Design review of the part shown in the three views and the two pictorial views. Dimensions are in mm from the part's minimum x, y and z. Coordinates: 2 decimals unless noted, no trailing zeros. Loops run counter-clockwise (first coordinate to the right, second up) from the corner with the lowest first, then second, coordinate; pieces in that order, holes last. Notation, with made-up numbers: M 41,-37 L 73,-37 A20 ccw 73,-1 Z; hole C 49.5,41.5 d8. An arc over 180 degrees is marked long. Answer as a JSON object with one key per item and string values. Group by question number.
Item 1: Wall thickness on L1, parallel to X at y = 1.7, z = 3; L2, parallel to X at y = 1.55, z = 3.5; L3, parallel to X at y = 0.4, z = 9: over which ranges is each line inside the solid? List them lowest first. Write a range as from..to.
Item 2: Add section D-D (y = 0.9). State the section outline as (x, z) points.
Item 3: Add section B-B (z = 7). State the section outline as (x, y) points (3 decimals), then the cut area to 3 significant figures.
Item 4: Insertion check: pin 1 (1.8 mm diameter, centred on x = 3, z = 3, fed in from -Y); pin 2 (6 mm diameter, centred on x = 4, z = 2.5, fed in from -Y). Each pin has a flat end and moves straight along its axis. Give the tip position at first contact, or say it passes through.
Item 5: Add section C-C (x = 17). State the section outline as (y, z) points, then the cut area to 3 significant figures.
Item 6: Add section A-A (y = 3.3). State the section outline as (x, z) points, then the cut area to 3 significant figures.
Item 7: Mouldability with a two-part tool opening along Z and no side actions: class the marked faces 1, 2, 3 and 4 as +Z half, -Z half, draft (parallel to the pull), parting line (faces both ways), or undercut.
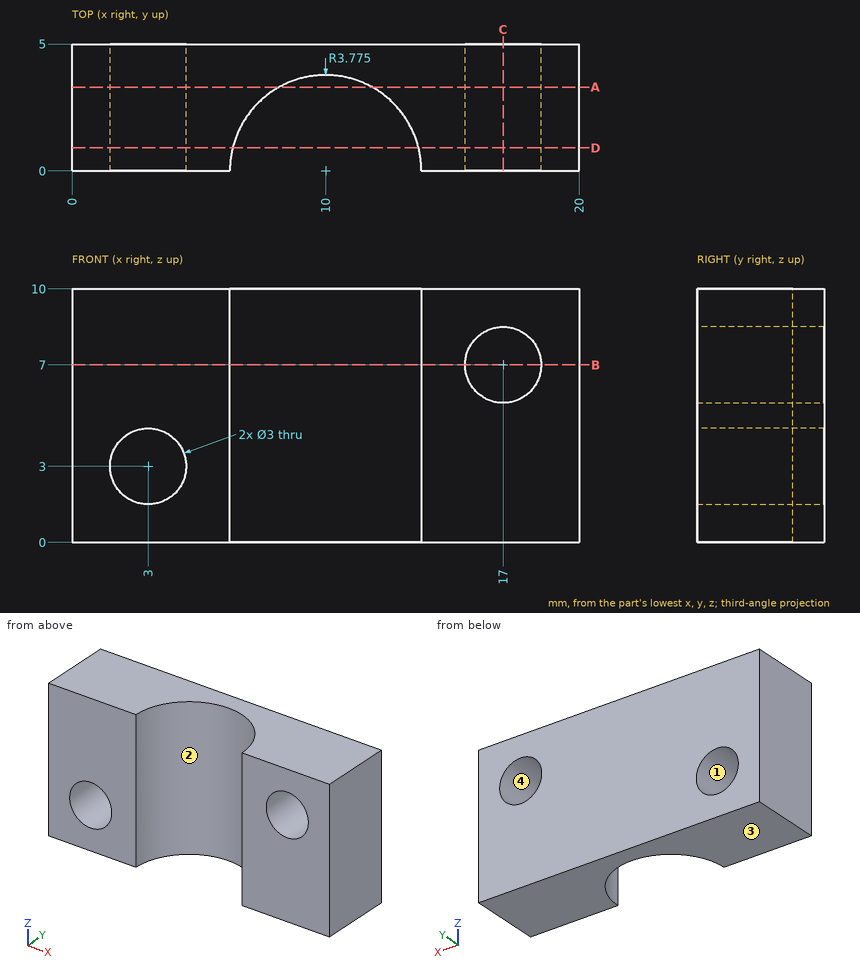
From the geometry:
{
 "1": {"L1": "x = 0..1.5, 4.5..6.63, 13.37..20", "L2": "x = 0..1.59, 4.41..6.56, 13.44..20", "L3": "x = 0..6.25, 13.75..20"},
 "2": {"outline": "M 0,0 L 6.33,0 L 6.33,10 L 0,10 Z; M 13.67,0 L 20,0 L 20,10 L 13.67,10 Z; hole C 3,3 d3; hole C 17,7 d3"},
 "3": {"outline": "M 0,0 L 6.225,0 A3.775 cw 13.775,0 L 15.5,0 L 15.5,5 L 0,5 Z; M 18.5,0 L 20,0 L 20,5 L 18.5,5 Z", "area": "62.6 mm²"},
 "4": {"pin 1": "passes through", "pin 2": "stops at y = 0"},
 "5": {"outline": "M 0,0 L 5,0 L 5,5.5 L 0,5.5 Z; M 0,8.5 L 5,8.5 L 5,10 L 0,10 Z", "area": "35.0 mm²"},
 "6": {"outline": "M 0,0 L 8.17,0 L 8.17,10 L 0,10 Z; M 11.83,0 L 20,0 L 20,10 L 11.83,10 Z; hole C 3,3 d3; hole C 17,7 d3", "area": "149 mm²"},
 "7": {"face 1": "undercut", "face 2": "draft", "face 3": "-Z half", "face 4": "undercut"}
}
